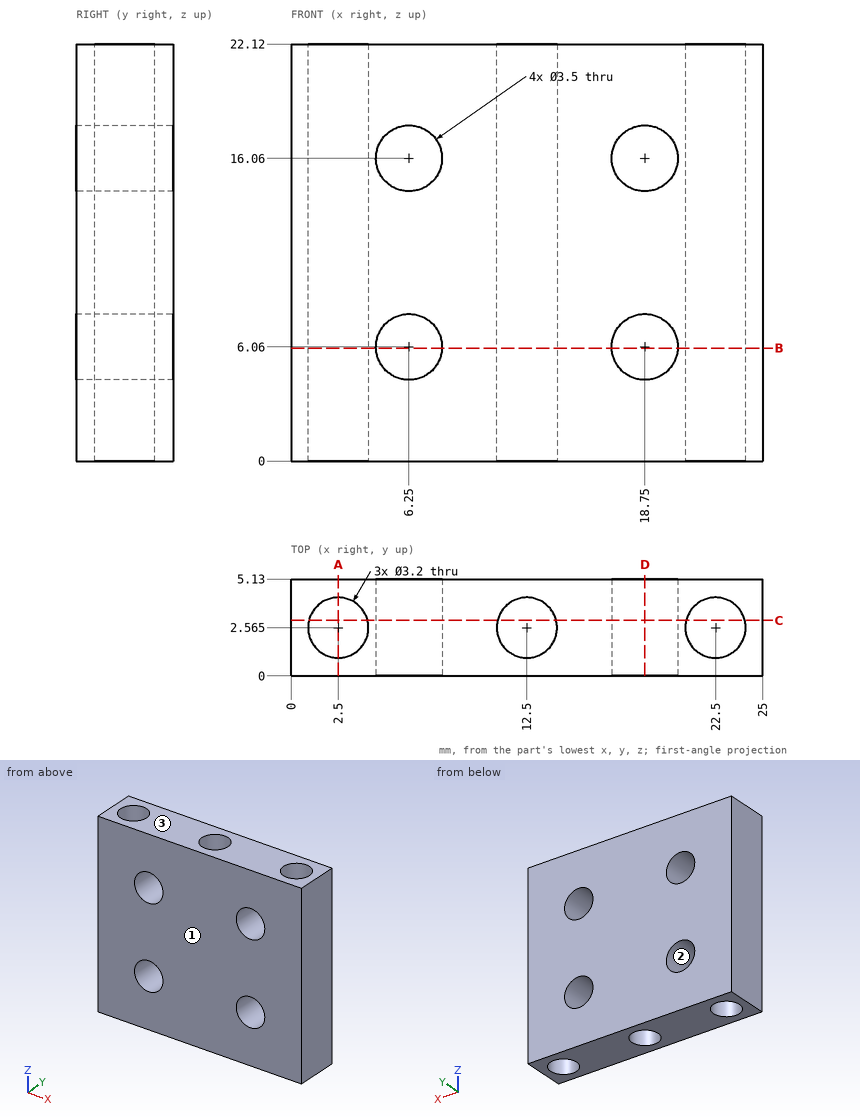
Input: dimensioned drawing with shaded views. Units: mm. Origin: part minimum x, y, z. Give positions to 0.01 mm unless a question says otherwise; leave off trailing zeros. Order: outer loops, then holes, each group sorted by start corner. A loop starts at its lowest first (then second) coordinate and runs counter-clockwise, first axis right, second up.
(1) Pull-direction query (Z, two-part tool) for the marked faces 1, 2 and 3; classes: +Z half, -Z half, draft (parallel to the pull), parting line (faces both ways), or undercut.
(2) Material intervals for line 1 along Y through (x, z) = (22.5, 7.25) (3 decimals); line 2 along X through (y, z) = (2.4, 6.5); line 3 along X through (y, z) = (1.2, 6), sorted ascending.
(3) Section query B-B (z = 6). Return the cut outline in (x, y) (3 decimals), plus the area to 3 significant figures.
(4) Section query C-C (y = 2.95). Return the cut outline in (x, z), plus the area to 3 significant figures.
(5) Section query D-D (x = 18.75). Return the cut outline in (y, z), plus the area to 3 significant figures.
(6) Section query A-A (x = 2.5). Return the cut outline in (y, z) (3 decimals), plus the area to 3 significant figures.
Outcome:
1. face 1: draft
1. face 2: undercut
1. face 3: +Z half
2. line 1: y = 0 to 0.965, 4.165 to 5.13
2. line 2: x = 0 to 0.91, 4.09 to 4.56, 7.94 to 10.91, 14.09 to 17.06, 20.44 to 20.91, 24.09 to 25
2. line 3: x = 0 to 1.67, 3.33 to 4.5, 8 to 11.67, 13.33 to 17, 20.5 to 21.67, 23.33 to 25
3. outline: (0, 0) - (4.501, 0) - (4.501, 5.13) - (0, 5.13) - close; (7.999, 0) - (17.001, 0) - (17.001, 5.13) - (7.999, 5.13) - close; (20.499, 0) - (25, 0) - (25, 5.13) - (20.499, 5.13) - close; hole circle Ø3.2 at (2.5, 2.565); hole circle Ø3.2 at (12.5, 2.565); hole circle Ø3.2 at (22.5, 2.565)
3. area: 68.2 mm2
4. outline: (0, 0) - (0.95, 0) - (0.95, 22.12) - (0, 22.12) - close; (4.05, 0) - (10.95, 0) - (10.95, 22.12) - (4.05, 22.12) - close; (14.05, 0) - (20.95, 0) - (20.95, 22.12) - (14.05, 22.12) - close; (24.05, 0) - (25, 0) - (25, 22.12) - (24.05, 22.12) - close; hole circle Ø3.5 at (6.25, 6.06); hole circle Ø3.5 at (6.25, 16.06); hole circle Ø3.5 at (18.75, 6.06); hole circle Ø3.5 at (18.75, 16.06)
4. area: 308 mm2
5. outline: (0, 0) - (5.13, 0) - (5.13, 4.31) - (0, 4.31) - close; (0, 7.81) - (5.13, 7.81) - (5.13, 14.31) - (0, 14.31) - close; (0, 17.81) - (5.13, 17.81) - (5.13, 22.12) - (0, 22.12) - close
5. area: 77.6 mm2
6. outline: (0, 0) - (0.965, 0) - (0.965, 22.12) - (0, 22.12) - close; (4.165, 0) - (5.13, 0) - (5.13, 22.12) - (4.165, 22.12) - close
6. area: 42.7 mm2
